Build history of the part. All positions in model axes, mm. A direction names the side the tool comes from. Give positions to 0.01 mm unless a question says otherwise; leave off trailing zeros. Loops run counter-clockwise (first coordinate to the right, second up) from the corner with the lowest first, then second, coordinate; pieces in that order, holes last. Notation, with made-up numbers: M 79.25,61 L 107.25,61 A31 cw 107.25,91 Z; hole C 62,8.25 d5. An arc over 180 degrees is marked long. Answer as a JSON object with one key per item and string values. Group by question number.
1. Slice it at C-C (x = 55.5). List the corners of the cut face in (y, z), then the cut area to 3 significant figures.
2. Slice it at A-A (x = 13). List the corners of the cut face in (y, z).
3. Drill centre lines: line 1 along X through (y, z) = (-17, 10); line 2 along X through (y, z) = (22.5, 9.5); line 3 along Y through (x, z) = (17, 12). Where is each one in solid material? Low to high. Write a range as [from, to].
4. 3-axis set-ups, long thin cutter, end or side, ignore diameter. For faces 5 (the face through (-41.068, 1.776, 5.133)), 6 (the face through (21.7, -24.95, 6.41)), 7 (the face through (-4.463, -32.533, 6.409)), 8 (the face through (-48.709, 46, 6)): which of +Z, -Z, +X, -X, +Y, -Y reach the whole face in a straight line?
5. Mould opens along Y. For faces 1 (the face through (-61.54, 39.42, 6.41)), 2 (the face through (14.043, 11.901, 1.014)), 3 (the face through (-29, 11, 0)), 4 (the face through (-35.57, 34.024, 6.355)) say: released by +Y, released by -Y, zero draft, split by the parting line, or undercut.
6. Drop flat-ended pins along their axis: pin 1 Ø1 at (x, z) = (10.5, 7.5) entering from -Y; pin 2 Ø1.5 at (x, y) = (17, -1.5) entering from +Z; pin 3 Ø5.5 at (y, z) = (21.5, 7.5) entering from +X. Give the stop position or say it passes through.
7. Slice it at B-B (y = 18.5). List the corners of the cut face in (x, z), then the cut area to 3 significant figures.
8. Slice it at D-D (x = 31). List the corners of the cut face in (y, z).
from build123d import *

# Parameters (mm, degrees)
F1_DEPTH  = 13
F2_R      = 16.193977
F3_DEPTH  = 13
F4_DEPTH  = 11
F9_R      = 7.442365
F10_DEPTH = 126.005636


with BuildPart() as f1:
    # F0 (on Top) → F1 (new body)
    with BuildSketch(Plane.XY):
        Polygon((-32.077711, -60.813792), (-8.803713, -31.388912), (0, -33.708788), (11.301869, -31.58224), (18.64814, -27.909102), (24.834473, -21.916091), (60.792536, 23.708114), (65.238968, 32.021001), (64.06498, 41.530453), (62.238194, 43.600813), (58.462832, 45.184027), (53.104255, 46.280101), (46.771396, 46.280101), (45.188177, 51.151533), (39.707817, 56.75368), (-42.984739, 54.926891), (-46.029385, 52.856531), (-48.708674, 47.376171), (-48.708674, 43.844383), (-56.259394, 42.74831), (-60.278326, 41.165095), (-62.835827, 37.633304), (-63.523754, 34.105126), (-59.529565, -59.653856), (-57.749115, -60.001009), (-43.858236, -62.709465), align=None)
    extrude(amount=F1_DEPTH)

    # F2 (on face) → F3 (cut, through all)
    with BuildSketch(Plane.XY.offset(13)):
        with Locations((-1.402867, 7.036958)):
            Circle(F2_R)
    extrude(amount=-F3_DEPTH, mode=Mode.SUBTRACT)

    # F2 (on face) → F4 (cut)
    with BuildSketch(Plane.XY.offset(13)):
        with BuildLine():
            ThreePointArc((-27.557551, -3.949325), (4.20068, -20.772503), (26.965529, 7.036958))
            ThreePointArc((26.965529, 7.036958), (11.817696, 32.136413), (-17.448869, 30.431225))
            ThreePointArc((-17.448869, 30.431225), (-28.619223, 15.0392), (-27.557551, -3.949325))
        make_face()
        with Locations((-1.402867, 7.036958)):
            Circle(F2_R, mode=Mode.SUBTRACT)
        with BuildLine():
            ThreePointArc((-27.557551, -3.949325), (-28.619223, 15.0392), (-17.448869, 30.431225))
            Line((-17.448869, 30.431225), (-54.205403, 37.718657))
            Line((-54.205403, 37.718657), (-54.205403, 7.342626))
            Line((-54.205403, 7.342626), (-27.557551, -3.949325))
        make_face()
    extrude(amount=-F4_DEPTH, mode=Mode.SUBTRACT)

    # F9 (on face) → F10 (cut, through all)
    with BuildSketch(Plane(origin=(12.679749, 47.321467, 0), x_dir=(0.965926, -0.258819, 0), z_dir=(-0.258819, -0.965926, 0))):
        with Locations((-38.978635, 13)):
            Circle(F9_R)
    extrude(amount=F10_DEPTH, mode=Mode.SUBTRACT)


solid = f1.part
Established:
{
 "1": {"outline": "M 16.99,0 L 45.79,0 L 45.79,13 L 16.99,13 Z", "area": "374 mm^2"},
 "2": {"outline": "M -30.73,0 L -0.37,0 L -0.37,2 L -17.4,2 L -17.4,13 L -30.73,13 Z; M 14.44,0 L 56.16,0 L 56.16,13 L 31.48,13 L 31.48,2 L 14.44,2 Z"},
 "3": {"line 1": "x = [-61.35, -51.96], [-37.86, -16.47], [13.66, 28.71]", "line 2": "x = [-63.03, -54.21], [22.38, 59.84]", "line 3": "y = [-28.73, -14.55], [28.63, 56.25]"},
 "4": {"face 5": "+Z", "face 6": "+Z, -Z, +X, -Y", "face 7": "+Z, -Z, -Y", "face 8": "+Z, -Z, -X, +Y"},
 "5": {"face 1": "released by +Y", "face 2": "undercut", "face 3": "zero draft", "face 4": "undercut"},
 "6": {"pin 1": "stops at y = -31.83", "pin 2": "stops at z = 2", "pin 3": "stops at x = 61.08"},
 "7": {"outline": "M -62.86,0 L -12.84,0 L -12.84,2 L -54.21,2 L -54.21,13 L -62.86,13 Z; M 10.04,0 L 56.69,0 L 56.69,13 L 24.55,13 L 24.55,2 L 10.04,2 Z", "area": "642 mm^2"},
 "8": {"outline": "M -14.09,0 L 56.56,0 L 56.56,13 L -14.09,13 Z"}
}
